Here's how the part is built. I have some questions about the finished solid (model axes, mm). A direction names the side the tool comes from. Coordinates: 2 decimals unless noted, no trailing zeros. Write each loop counter-clockwise with the first axis right and the second up, starting at its lowest first coordinate (ties: lowest second). Pieces come first, ordered by that corner, then holes. Notation, with made-up numbers: M 40,-9 L 90,-9 A17 ccw 90,-3 Z; hole C -8,35 d5. An arc over 180 degrees is marked long. Use one line per item in the form item = value. Start each with the question number.
1. I want a section at A-A, the plane x = 15.5. List the corners of the cut face in (y, z) for me (3 decimals), plus the area to 3 significant figures.
2. Please list where these lines run through material, in increasing order: line 1 along Y through (x, z) = (18.25, 0) (3 decimals); line 2 along X through (y, z) = (-2.75, 2.5); line 3 along Z through (x, y) = (27, -1). Write a range as [from, to].
3. I want a section at B-B, the plane y = 0. List the corners of the cut face in (x, z) for me (3 decimals), plus the area to 3 significant figures.
4. I'm going to push flat-ended pins straight in: pin 1 Ø2 at (x, z) = (13, 1) entering from +Y; pin 2 Ø1.5 at (y, z) = (2.5, 2) entering from +X; pin 3 Ø6 at (x, y) = (21, 1.5) entering from +Z (3 decimals). Where does each tip first touch, or does it pass through?
5. I want a section at D-D, the plane x = 26. List the corners of the cut face in (y, z) for me, plus the area to 3 significant figures.
6. On a 3-axis mill with a long thin cutter (end or side, diameter ignored), from which of +Z, -Z, +X, -X, +Y, -Y can I reach the whole of each face in a straight line? I mean faces 1 (the face through (21.3, -2.1, -1.4)), 2 (the face through (31.8, 0, 0)). Say none if no direction works.
7. I want a section at C-C, the plane z = 0. List the corners of the cut face in (x, y) for me (3 decimals).
8. Thinking about a two-plate mould opening in Y: for faces 3 (the face through (6, 6.6, 0)), 4 (the face through (6, -6.6, 0)), 5 (the face through (6, 0, 3.5)), 6 (the face through (16.86, 2.23, 0.29)), which applies, released by +Y, released by -Y, zero draft, split by the parting line, or undercut?
Autodesk Inventor part; units mm, degrees
ref_plane "YZ Plane" through (0, 0, 0) normal (1, 0, 0) x (0, 1, 0)
ref_plane "XZ Plane" through (0, 0, 0) normal (0, 1, 0) x (-1, 0, 0)
ref_plane "XY Plane" through (0, 0, 0) normal (0, 0, 1) x (1, 0, 0)
sketch "Sketch1" plane through (0, 0, 0) normal (1, 0, 0) x (0, 1, 0)
  line L0 (6.6, 3.5) -> (-6.6, 3.5)
  line L1 (-6.6, 3.5) -> (-6.6, -3.5)
  line L2 (-6.6, -3.5) -> (6.6, -3.5)
  line L3 (6.6, -3.5) -> (6.6, 3.5)
  line L4 (6.6, 3.5) -> (-6.6, -3.5) construction
  line L5 (-6.6, 3.5) -> (6.6, -3.5) construction
  point P0 (0, 0)
  dimension "d0" = 13.2
  dimension "d1" = 7
extrude "Extrusion1" add sketch "Sketch1" along normal blind 12.3
sketch "Sketch2" plane through (12.3, 0, 0) normal (1, 0, 0) x (0, 0, -1)
  circle A0 centre (0, 0) radius 3.175
  dimension "d4" = 6.35
extrude "Extrusion2" add sketch "Sketch2" along normal blind 9
sketch "Sketch3" plane through (21.3, 0, 0) normal (1, 0, 0) x (0, 0, -1)
  circle A0 centre (0, 0) radius 2.25
  dimension "d7" = 4.5
extrude "Extrusion3" cut sketch "Sketch3" against normal blind 9
sketch "Sketch4" plane through (21.3, 0, 0) normal (1, 0, 0) x (0, 0, -1)
  circle A0 centre (0, 0) radius 1.5
  dimension "d10" = 3
extrude "Extrusion4" add sketch "Sketch4" along normal blind 10.5
sketch "Sketch5" plane through (21.3, 0, 0) normal (-1, 0, 0) x (0, 0, 1)
  circle A0 centre (0, 0) radius 1.5
extrude "Extrusion5" add sketch "Sketch5" along normal up to surface (9 mm away)
thread "Thread1"
properties part number "APEM_5236CDB" material "Stainless Steel"
Answer list:
q1.outline = C 0,0 d6.35; C 0,0 d3; hole C 0,0 d4.5
q1.area = 22.8 mm²
q2.line_1 = [-3.175, -2.25], [-1.5, 1.5], [2.25, 3.175]
q2.line_2 = [0, 12.3]
q2.line_3 = [-1.12, 1.12]
q3.outline = M 0,-3.5 L 12.3,-3.5 L 12.3,-3.175 L 21.3,-3.175 L 21.3,-2.25 L 12.3,-2.25 L 12.3,-1.5 L 31.8,-1.5 L 31.8,1.5 L 12.3,1.5 L 12.3,2.25 L 21.3,2.25 L 21.3,3.175 L 12.3,3.175 L 12.3,3.5 L 0,3.5 Z
q3.area = 161 mm²
q4.pin_1 = 6.6
q4.pin_2 = 21.3
q4.pin_3 = 3.175
q5.outline = C 0,0 d3
q5.area = 7.07 mm²
q6.face_1 = +X
q6.face_2 = +Z, -Z, +X, +Y, -Y
q7.outline = M 0,-6.6 L 12.3,-6.6 L 12.3,-3.175 L 21.3,-3.175 L 21.3,-2.25 L 12.3,-2.25 L 12.3,-1.5 L 31.8,-1.5 L 31.8,1.5 L 12.3,1.5 L 12.3,2.25 L 21.3,2.25 L 21.3,3.175 L 12.3,3.175 L 12.3,6.6 L 0,6.6 Z
q8.face_3 = released by +Y
q8.face_4 = released by -Y
q8.face_5 = zero draft
q8.face_6 = undercut
